Can you work these out from the model? Positions are in its coordinate system, mm. A direction names the side the tool comes from. Give positions to 0.01 mm unless a question says otherwise; leave off trailing zeros. Loops run counter-clockwise (first coordinate to the right, second up) from the corner with the lowest first, then second, coordinate; pieces in that order, holes last. Notation, with made-up numbers: (-36, 78) -> (-18, 78) arc R20 ccw to (-18, 117) -> close; hole circle Ø5 at (39.25, 87). An arc over 180 degrees is marked (long way). Return JSON: item names as keys, results as strings. Group by question number.
Q1. Suppose I cut it at D-D, the plane x = -41.5. Please give me the cut outline in (y, z), and give its area (3 significant figures).
Q2. Will these pins go through, and if not, where does the flat tip stop? pin 1 (1.5 mm diameter, centred on x = 2, y = -47, fed in from -Z); pin 2 (6 mm diameter, centred on x = -6.5, z = 31, fed in from -Y) (1 decimal); pin 3 (8 mm diameter, centred on y = 37.5, z = 25, fed in from -X); pin 4 (10 mm diameter, centred on y = 35, z = 25, fed in from -X).
Q3. Which directions (+Z, -Z, +X, -X, +Y, -Y) give clear straight access to the entire face, cutting with the end or side of a thin tool? Please do faces 1 (the flat face through (44.2, -18.3, 50)), 2 (the flat face through (0, -48, 10)), 3 (the flat face through (-1, 1, 2.5)).
Q4. Thinking about a two-plate mould opening in Y: for faces 4 (the cylindrical face through (47.69, 15.02, 24.65)), 5 (the flat face through (0, 48, 10)), 6 (the cylindrical face through (45.307, 14.268, 25.918)), which applies, pulls with the +Y half, pulls with the -Y half, needs draft (parallel to the pull), parting line crosses it, or undercut?
Q5. Suppose I cut it at A-A, the plane z = 12.5. Please give me the cut outline in (x, y), and give its area (3 significant figures).
Q6. Suppose I cut it at B-B, the plane x = 0. Please give me the cut outline in (y, z).
Q7. Suppose I cut it at C-C, the plane y = 0. Please give me the cut outline in (x, z), and give its area (4 significant figures).
Q8. I need wall thicknesses on line 1 along Y through (x, z) = (0, 40.5); line 2 along Z through (x, y) = (40, 6.5); line 3 along Y through (x, z) = (17.5, 7). Which ranges of each line are inside material? Lowest first, please. Write a range as [from, to].
```python
from build123d import *

# Parameters (mm, degrees)
F0_R          = 50
F1_DEPTH      = 50
F2_T          = -2.5
F3_W          = 30
F3_H          = 25
F4_DEPTH      = 50.001
F4_DEPTH_BACK = 50.001


with BuildPart() as f1:
    # F0 (on Top) → F1 (new body)
    with BuildSketch(Plane.XY):
        Circle(F0_R)
    extrude(amount=F1_DEPTH)

    # F2
    f2_openings = [f1.faces().sort_by_distance(p)[0] for p in [
        (0, 0, 50),
    ]]
    offset(amount=F2_T, openings=f2_openings)

    # F3 (on Front) → F4 (cut, two sides)
    with BuildSketch(Plane.XZ) as f4_sk:
        with Locations((0, 22.5)):
            Rectangle(F3_W, F3_H)
    extrude(amount=F4_DEPTH, mode=Mode.SUBTRACT)
    extrude(f4_sk.sketch, amount=-F4_DEPTH_BACK, mode=Mode.SUBTRACT)


solid = f1.part
```
Ans:
{
 "1": {"outline": "(-27.89, 0) -> (27.89, 0) -> (27.89, 50) -> (23.11, 50) -> (23.11, 2.5) -> (-23.11, 2.5) -> (-23.11, 50) -> (-27.89, 50) -> close", "area": "594 mm^2"},
 "2": {"pin 1": "stops at z = 0", "pin 2": "passes through", "pin 3": "stops at x = -37.12", "pin 4": "stops at x = -40"},
 "3": {"face 1": "+Z, +X, -X, +Y, -Y", "face 2": "+Y, -Y", "face 3": "+Z"},
 "4": {"face 4": "parting line crosses it", "face 5": "needs draft", "face 6": "undercut"},
 "5": {"outline": "(-15, -47.7) -> (-15, -45.07) arc R47.5 cw to (-15, 45.07) -> (-15, 47.7) arc R50 ccw to start; (15, -47.7) arc R50 ccw to (15, 47.7) -> (15, 45.07) arc R47.5 cw to (15, -45.07) -> close", "area": "613 mm^2"},
 "6": {"outline": "(-50, 0) -> (50, 0) -> (50, 10) -> (47.5, 10) -> (47.5, 2.5) -> (-47.5, 2.5) -> (-47.5, 10) -> (-50, 10) -> close; (-50, 35) -> (-47.5, 35) -> (-47.5, 50) -> (-50, 50) -> close; (47.5, 35) -> (50, 35) -> (50, 50) -> (47.5, 50) -> close"},
 "7": {"outline": "(-50, 0) -> (50, 0) -> (50, 50) -> (47.5, 50) -> (47.5, 2.5) -> (-47.5, 2.5) -> (-47.5, 50) -> (-50, 50) -> close", "area": "487.5 mm^2"},
 "8": {"line 1": "y = [-50, -47.5], [47.5, 50]", "line 2": "z = [0, 2.5]", "line 3": "y = [-46.84, -44.16], [44.16, 46.84]"}
}
